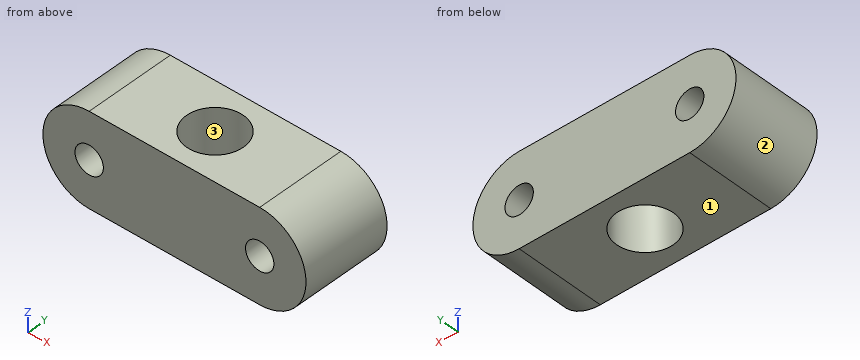
```python
from build123d import *

# Parameters (mm, degrees)
SKETCH1_R           = 6
BOSS_EXTRUDE1_DEPTH = 38
SKETCH3_R           = 12
CUT_EXTRUDE2_DEPTH  = 98


with BuildPart() as part:
    # Sketch1 → Boss-Extrude1 (new body)
    with BuildSketch(Plane(origin=(0, 0, 0), x_dir=(1, 0, 0), z_dir=(0, 1, 0))):
        with BuildLine():
            Line((0, 19.577833845), (72.128861533, 19.577833845))
            ThreePointArc((72.128861533, 19.577833845), (91.706695377, 0), (72.128861533, -19.577833845))
            Line((72.128861533, -19.577833845), (0, -19.577833845))
            ThreePointArc((0, -19.577833845), (-19.577833845, 0), (0, 19.577833845))
        make_face()
        Circle(SKETCH1_R, mode=Mode.SUBTRACT)
        with Locations((72.128861533, 0)):
            Circle(SKETCH1_R, mode=Mode.SUBTRACT)
    extrude(amount=BOSS_EXTRUDE1_DEPTH)

    # Sketch3 → Cut-Extrude2 (cut)
    with BuildSketch(Plane.XY.offset(19.577833845)):
        with Locations((36.064430766, 19)):
            Circle(SKETCH3_R)
    extrude(amount=-CUT_EXTRUDE2_DEPTH, mode=Mode.SUBTRACT)


solid = part.part
```
Input: part model. Units: mm. Frame: model coordinates. Face numbers are marked on the shaded views. Coordinates: 2 decimals unless noted, no trailing zeros. Write each loop counter-clockwise with the first axis right and the second up, starting at its lowest first coordinate (ties: lowest second). Pieces come first, ordered by that corner, then holes. Notation, with made-up numbers: (-4.5, 34) -> (-0.5, 34) arc R5 ccw to (-0.5, 41) -> close; hole circle Ø7 at (-27.75, -39). An arc over 180 degrees is marked (long way). Answer as a JSON object with one key per item and string values.
1. Section B-B on z = 0. Return the cut outline in (x, y).
Result set:
{"outline": "(-19.58, 0) -> (-6, 0) -> (-6, 38) -> (-19.58, 38) -> close; (6, 0) -> (66.13, 0) -> (66.13, 38) -> (6, 38) -> close; (78.13, 0) -> (91.71, 0) -> (91.71, 38) -> (78.13, 38) -> close; hole circle Ø24 at (36.06, 19)"}
2. Section A-A on y = 19. Return the cut outline in (x, z), then the cut area to 3 significant figures.
Result set:
{"outline": "(0, -19.58) -> (24.06, -19.58) -> (24.06, 19.58) -> (0, 19.58) arc R19.58 ccw to start; (48.06, -19.58) -> (72.13, -19.58) arc R19.58 ccw to (72.13, 19.58) -> (48.06, 19.58) -> close; hole circle Ø12 at (0, 0); hole circle Ø12 at (72.13, 0)", "area": "2,860 mm2"}
3. First-contact query: P1, Ø4, axis at y = 4.5, z = -8, coming from the -X side; P2, Ø10, axis at x = 7.5, z = -8.5, coming from the -Y side; P3, Ø3, axis at x = 77.5, y = 17.5, coming from the -Z side. Flat tips, straight axial feed; report the tip coordinate or a pass-through.
Result set:
{"P1": "stops at x = -18.64", "P2": "stops at y = 0", "P3": "stops at z = -19.19"}
4. Material intervals for line 1 (X direction, y = 15, z = 0); line 2 (X direction, y = 10.5, z = 0); line 3 (Z direction, x = 68.5, y = 19.5), sorted ascending. Write a range as from..to.
Result set:
{"line 1": "x = -19.58..-6, 6..24.75, 47.38..66.13, 78.13..91.71", "line 2": "x = -19.58..-6, 6..27.59, 44.53..66.13, 78.13..91.71", "line 3": "z = -19.58..-4.78, 4.78..19.58"}
5. Mould query, pull axis X, two halves, no side actions, for the marked faces 1, 2 and 3. Classes: released by +X, released by -X, zero draft, split by the parting line, or undercut.
Result set:
{"face 1": "zero draft", "face 2": "released by -X", "face 3": "undercut"}
6. Section C-C on x = 34. Return the cut outline in (y, z), then the cut area to 3 significant figures.
Result set:
{"outline": "(0, -19.58) -> (7.18, -19.58) -> (7.18, 19.58) -> (0, 19.58) -> close; (30.82, -19.58) -> (38, -19.58) -> (38, 19.58) -> (30.82, 19.58) -> close", "area": "562 mm2"}
7. Section D-D on z = -4.5. Return the cut outline in (x, y).
Result set:
{"outline": "(-19.05, 0) -> (-3.97, 0) -> (-3.97, 38) -> (-19.05, 38) -> close; (3.97, 0) -> (68.16, 0) -> (68.16, 38) -> (3.97, 38) -> close; (76.1, 0) -> (91.18, 0) -> (91.18, 38) -> (76.1, 38) -> close; hole circle Ø24 at (36.06, 19)"}
